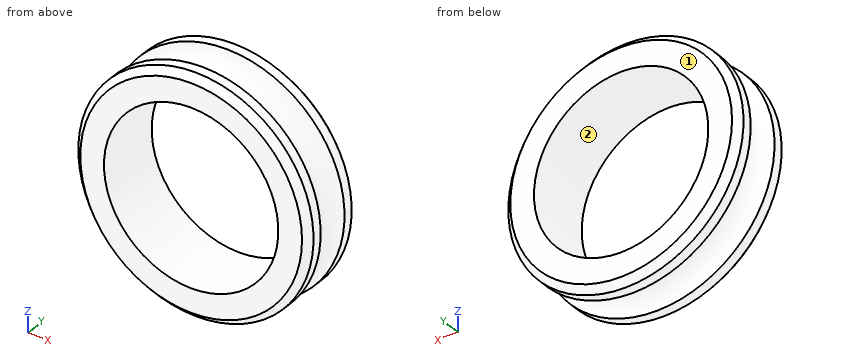
from build123d import *

# Parameters (mm, degrees)
SKETCH1_R                 = 17.5
SKETCH1_R_2               = 12.975
CORPO_EXTERNO_35_10_DEPTH = 10
CHANFROS_1_45_SIZE        = 1


with BuildPart() as part:
    # Sketch1 → Corpo Externo Ø35×10 (new body)
    with BuildSketch(Plane(origin=(0, 0, 0), x_dir=(1, 0, 0), z_dir=(0, 1, 0))):
        with Locations(Location((0, 0, 0), (0, 0, 270))):
            Circle(SKETCH1_R)
        with Locations(Location((0, 0, 0), (0, 0, 270))):
            Circle(SKETCH1_R_2, mode=Mode.SUBTRACT)
    extrude(amount=CORPO_EXTERNO_35_10_DEPTH)

    # Chanfros 1×45°
    chanfros_1_45_edges = [part.edges().sort_by_distance(p)[0] for p in [
        (0, 10, -17.5),
        (0, 0, -17.5),
    ]]
    chamfer(chanfros_1_45_edges, length=CHANFROS_1_45_SIZE)

    # Sketch2 → Canal (revolve, cut)
    with BuildSketch(Plane.XY, mode=Mode.PRIVATE) as canal_sk:
        with BuildLine():
            ThreePointArc((-17.5, 7.5), (-15, 5), (-17.5, 2.5))
            Line((-17.5, 2.5), (-17.5, 7.5))
        make_face()
    revolve(canal_sk.sketch.rotate(Axis((0, 0, 0), (0, 1, 0)), 270), axis=Axis((0, 0, 0), (0, 1, 0)), mode=Mode.SUBTRACT)


solid = part.part
Design review of the part built by this model. Coordinates are the model's own, in mm. Face numbers are marked on the shaded views. Give positions to 0.01 mm unless a question says otherwise; leave off trailing zeros. Loops run counter-clockwise (first coordinate to the right, second up) from the corner with the lowest first, then second, coordinate; pieces in that order, holes last. Notation, with made-up numbers: M -7.75,22 L -3.75,22 A23 cw -3.75,34 Z; hole C 79,36.25 d5. An arc over 180 degrees is marked long. Answer as a JSON object with one key per item and string values.
Item 1: Mouldability with a two-part tool opening along X and no side actions: class the marked faces 1 and 2 as pulls with the +X half, pulls with the -X half, needs draft (parallel to the pull), parting line crosses it, or undercut.
Output values:
{"face 1": "needs draft", "face 2": "undercut"}
Item 2: We need section C-C (y = 0.5). State the section outline as (x, z) points (3 decimals).
Output values:
{"outline": "C 0,0 d34; hole C 0,0 d25.95"}
Item 3: We need section B-B (x = 0). State the section outline as (y, z) points (3 decimals).
Output values:
{"outline": "M 0,-16.5 L 1,-17.5 L 2.5,-17.5 A2.5 cw 7.5,-17.5 L 9,-17.5 L 10,-16.5 L 10,-12.975 L 0,-12.975 Z; M 0,12.975 L 10,12.975 L 10,16.5 L 9,17.5 L 7.5,17.5 A2.5 cw 2.5,17.5 L 1,17.5 L 0,16.5 Z"}
Item 4: We need section A-A (z = 0). State the section outline as (x, y) points (3 decimals).
Output values:
{"outline": "M -17.5,1 L -16.5,0 L -12.975,0 L -12.975,10 L -16.5,10 L -17.5,9 L -17.5,7.5 A2.5 cw -17.5,2.5 Z; M 12.975,0 L 16.5,0 L 17.5,1 L 17.5,2.5 A2.5 cw 17.5,7.5 L 17.5,9 L 16.5,10 L 12.975,10 Z"}
Item 5: We need section D-D (y = 3). State the section outline as (x, z) points (3 decimals).
Output values:
{"outline": "C 0,0 d32; hole C 0,0 d25.95"}
Item 6: Wall thickness on line 1 along X through (y, z) = (8, 0) (3 decimals); line 2 along X through (y, z) = (2.25, -1); line 3 along Z through (x, y) = (-3, 1): over which ranges is each line inside the solid? List them lowest first.
Output values:
{"line 1": "x = -17.5 to -12.975, 12.975 to 17.5", "line 2": "x = -17.47 to -12.94, 12.94 to 17.47", "line 3": "z = -17.24 to -12.62, 12.62 to 17.24"}
Item 7: For P1, Ø1.5, axis at y = 2.5, z = -6, coming from the +X side; P2, Ø6, axis at y = 3.5, z = 12.5, coming from the -X side; P3, Ø5, axis at y = 8, z = -3.5, coming from the +X side, all flat-tipped, find the tip position at first contact; note any pin that passes through.
Output values:
{"P1": "stops at x = 16.69", "P2": "stops at x = -14.58", "P3": "stops at x = 17.47"}
